The listing builds one solid part. Answer for the finished solid, in the listing's coordinates (mm). A direction names the side the tool comes from. Coordinates: 2 decimals unless noted, no trailing zeros. Order: outer loops, then holes, each group sorted by start corner. A loop starts at its lowest first (then second) coordinate and runs counter-clockwise, first axis right, second up. Notation, with made-up numbers: (-14, -24.5) -> (21, -24.5) arc R17 ccw to (21, -7.5) -> close; hole circle Ø5 at (-20, -27.75). An arc over 180 degrees is marked (long way). Answer in a Markdown table with one row per item.
```python
from build123d import *

# Parameters (mm, degrees)
SKETCH1_R                = 37.5
BOSS_EXTRUDE1_DEPTH      = 12
SKETCH2_R                = 30
BOSS_EXTRUDE2_DEPTH      = 56
BOSS_EXTRUDE3_DEPTH      = 5
BOSS_EXTRUDE3_DEPTH_BACK = 1
SKETCH4_W                = 75
SKETCH4_H                = 15
SKETCH4_R                = 3.5
MOVE_FACE3_BY            = 10
MOVE_FACE3_2_BY          = 10
BOSS_EXTRUDE4_DEPTH      = 12
BOSS_EXTRUDE5_DEPTH      = 68
MOVE_START               = 42.5
MOVE_FACE1_OUTLINE_W     = 95
MOVE_FACE1_OUTLINE_H     = 83
MOVE_FACE1_OUTLINE_R     = 3.5
MOVE_FACE1_DEPTH         = 10
SKETCH11_W               = 95
SKETCH11_H               = 15
BOSS_EXTRUDE7_DEPTH      = 20
CUT_EXTRUDE1_DEPTH       = 103.720494547
CUT_EXTRUDE1_DEPTH_BACK  = 103.720494547
SKETCH12_R               = 2.5
SKETCH13_R               = 6.5
CUT_EXTRUDE2_DEPTH       = 5
MOVE_FACE2_BY            = 7
DELETEFACE1_START        = -20
DELETEFACE1_OUTLINE_W    = 95
DELETEFACE1_OUTLINE_H    = 8
DELETEFACE1_DEPTH        = 20
CUT_EXTRUDE3_DEPTH       = 103.359660059
CUT_EXTRUDE3_DEPTH_BACK  = 3
SKETCH15_R               = 2
CUT_EXTRUDE4_DEPTH       = 96.818839484
MOVE_FACE4_BY            = 20
SKETCH16_W               = 55
SKETCH16_H               = 35
CUT_EXTRUDE5_DEPTH       = 10
SKETCH17_W               = 20
SKETCH17_H               = 50
CUT_EXTRUDE6_DEPTH       = 5
SKETCH18_R               = 2
CUT_EXTRUDE7_DEPTH       = 114.535236825
SKETCH19_R               = 2.5
CUT_EXTRUDE8_DEPTH       = 114.781589028


# Read off the part's stored shape, not the designer's step: Move Face1, DeleteFace1
with BuildPart() as part:
    # Sketch1 → Boss-Extrude1 (new body)
    with BuildSketch(Plane(origin=(0, 0, 0), x_dir=(1, 0, 0), z_dir=(0, 1, 0))):
        with Locations(Location((0, 0, 0), (0, 0, 270))):
            Circle(SKETCH1_R)
    extrude(amount=BOSS_EXTRUDE1_DEPTH)

    # Sketch2 → Boss-Extrude2 (add)
    with BuildSketch(Plane(origin=(0, 12, 0), x_dir=(1, 0, 0), z_dir=(0, 1, 0))):
        with Locations(Location((0, 0, 0), (0, 0, 270))):
            Circle(SKETCH2_R)
    extrude(amount=BOSS_EXTRUDE2_DEPTH)


with BuildPart() as body_2:
    # Sketch4 → Boss-Extrude3 (new, two sides: drawn at the far end of the back side and taken through both)
    with BuildSketch(Plane.XY.offset(37.5).offset(-BOSS_EXTRUDE3_DEPTH_BACK)):
        with Locations((0, 75.5)):
            Rectangle(SKETCH4_W, SKETCH4_H)
        with Locations((0, 76)):
            Circle(SKETCH4_R, mode=Mode.SUBTRACT)
    extrude(amount=BOSS_EXTRUDE3_DEPTH + BOSS_EXTRUDE3_DEPTH_BACK)

    # Move Face3: a face moved outward by 10.0
    extrude(body_2.faces().sort_by_distance((-37.5, 75.5, 39.5))[0], amount=MOVE_FACE3_BY, dir=(-1, 0, 0))

    # Move Face3 2: a face moved outward by 10.0
    extrude(body_2.faces().sort_by_distance((37.5, 75.5, 39.5))[0], amount=MOVE_FACE3_2_BY, dir=(1, 0, 0))



with BuildPart() as body_3:
    # Sketch6 → Boss-Extrude4 (new body)
    with BuildSketch(Plane.XZ):
        with BuildLine():
            Line((42.5, 0), (37.5, 0))
            ThreePointArc((37.5, 0), (0, 37.5), (-37.5, 0))
            Line((-37.5, 0), (-42.5, 0))
            ThreePointArc((-42.5, 0), (0, 42.5), (42.5, 0))
        make_face()
    extrude(amount=-BOSS_EXTRUDE4_DEPTH)


with BuildPart() as body_2_1:
    add(body_2.part)

    add(body_3.part)  # Boss-Extrude5 merges body 3
    # Sketch7 → Boss-Extrude5 (add)
    with BuildSketch(Plane.XZ.offset(-68)):
        with BuildLine():
            Line((8.602325267, 36.5), (47.5, 36.5))
            Line((47.5, 36.5), (47.5, 42.5))
            Line((47.5, 42.5), (-47.5, 42.5))
            Line((-47.5, 42.5), (-47.5, 36.5))
            Line((-47.5, 36.5), (-8.602325267, 36.5))
            ThreePointArc((-8.602325267, 36.5), (0, 37.5), (8.602325267, 36.5))
        make_face()
    extrude(amount=BOSS_EXTRUDE5_DEPTH)

    # Move Face1 outline → Move Face1 (add)
    with BuildSketch(Plane.XY.offset(MOVE_START)):
        with Locations((0, 41.5)):
            Rectangle(MOVE_FACE1_OUTLINE_W, MOVE_FACE1_OUTLINE_H)
        with Locations((0, 76)):
            Circle(MOVE_FACE1_OUTLINE_R, mode=Mode.SUBTRACT)
    extrude(amount=MOVE_FACE1_DEPTH)

    # Sketch11 → Boss-Extrude7 (add)
    with BuildSketch(Plane.XZ):
        with Locations((0, 45)):
            Rectangle(SKETCH11_W, SKETCH11_H)
    extrude(amount=BOSS_EXTRUDE7_DEPTH)

    # Sketch12 → Cut-Extrude1 (cut, two sides: drawn at the far end of the back side and taken through both)
    with BuildSketch(Plane(origin=(0, 0, 37.5), x_dir=(-1, 0, 0), z_dir=(0, 0, -1)).offset(-CUT_EXTRUDE1_DEPTH_BACK)):
        with Locations((-15, 20)):
            Circle(SKETCH12_R)
        with Locations((15, 20)):
            Circle(SKETCH12_R)
        with Locations((-15, 50)):
            Circle(SKETCH12_R)
        with Locations((15, 50)):
            Circle(SKETCH12_R)
    extrude(amount=CUT_EXTRUDE1_DEPTH + CUT_EXTRUDE1_DEPTH_BACK, mode=Mode.SUBTRACT)

    # Sketch13 → Cut-Extrude2 (cut)
    with BuildSketch(Plane(origin=(0, 0, 36.5), x_dir=(-1, 0, 0), z_dir=(0, 0, -1))):
        with Locations((-15, 50)):
            Circle(SKETCH13_R)
        with Locations((15, 50)):
            Circle(SKETCH13_R)
        with Locations((-15, 20)):
            Circle(SKETCH13_R)
        with Locations((15, 20)):
            Circle(SKETCH13_R)
    extrude(amount=-CUT_EXTRUDE2_DEPTH, mode=Mode.SUBTRACT)

    # Move Face2: a face moved inward by 7.0
    extrude(body_2_1.faces().sort_by_distance((0, 31.294429556, 52.5))[0], amount=MOVE_FACE2_BY, dir=(0, 0, -1), mode=Mode.SUBTRACT)

    # DeleteFace1 outline → DeleteFace1 (cut)
    with BuildSketch(Plane(origin=(0, 0, 0), x_dir=(1, 0, 0), z_dir=(0, 1, 0)).offset(DELETEFACE1_START)):
        with Locations((0, -41.5)):
            Rectangle(DELETEFACE1_OUTLINE_W, DELETEFACE1_OUTLINE_H)
    extrude(amount=DELETEFACE1_DEPTH, mode=Mode.SUBTRACT)

    # Sketch14 → Cut-Extrude3 (cut, two sides: drawn at the far end of the back side and taken through both)
    with BuildSketch(Plane(origin=(0, 0, 36.5), x_dir=(-1, 0, 0), z_dir=(0, 0, -1)).offset(-CUT_EXTRUDE3_DEPTH_BACK)):
        Polygon((47.5, 0), (-42.5, 0), (-47.5, 0), (-47.5, 12), (-42.5, 12), (47.5, 12), align=None)
    extrude(amount=CUT_EXTRUDE3_DEPTH + CUT_EXTRUDE3_DEPTH_BACK, mode=Mode.SUBTRACT)

    # Sketch15 → Cut-Extrude4 (cut, through all)
    with BuildSketch(Plane(origin=(0, 0, 39.5), x_dir=(-1, 0, 0), z_dir=(0, 0, -1))):
        with Locations((44.5, 6)):
            Circle(SKETCH15_R)
        with Locations((-44.5, 6)):
            Circle(SKETCH15_R)
    extrude(amount=-CUT_EXTRUDE4_DEPTH, mode=Mode.SUBTRACT)

    # Move Face4: a face moved outward by 20.0
    extrude(body_2_1.faces().sort_by_distance((0, 83, 41))[0], amount=MOVE_FACE4_BY, dir=(0, 1, 0))

    # Sketch16 → Cut-Extrude5 (cut)
    with BuildSketch(Plane(origin=(0, 0, 36.5), x_dir=(-1, 0, 0), z_dir=(0, 0, -1))):
        with Locations((0, 85.5)):
            Rectangle(SKETCH16_W, SKETCH16_H)
    extrude(amount=-CUT_EXTRUDE5_DEPTH, mode=Mode.SUBTRACT)

    # Sketch17 → Cut-Extrude6 (cut)
    with BuildSketch(Plane(origin=(0, 0, 36.5), x_dir=(-1, 0, 0), z_dir=(0, 0, -1))):
        with Locations((37.5, 78)):
            Rectangle(SKETCH17_W, SKETCH17_H)
        with Locations((-37.5, 78)):
            Rectangle(SKETCH17_W, SKETCH17_H)
    extrude(amount=-CUT_EXTRUDE6_DEPTH, mode=Mode.SUBTRACT)

    # Sketch18 → Cut-Extrude7 (cut, through all)
    with BuildSketch(Plane(origin=(0, 0, 41.5), x_dir=(-1, 0, 0), z_dir=(0, 0, -1))):
        with Locations((-42.5, 58)):
            Circle(SKETCH18_R)
        with Locations((-42.5, 100)):
            Circle(SKETCH18_R)
        with Locations(Location((42.5, 100, 0), (0, 0, 180))):
            Circle(SKETCH18_R)
        with Locations(Location((42.5, 58, 0), (0, 0, 180))):
            Circle(SKETCH18_R)
    extrude(amount=-CUT_EXTRUDE7_DEPTH, mode=Mode.SUBTRACT)

    # Sketch19 → Cut-Extrude8 (cut, through all)
    with BuildSketch(Plane.XY.offset(45.5)):
        with Locations((0, 35)):
            Circle(SKETCH19_R)
    extrude(amount=-CUT_EXTRUDE8_DEPTH, mode=Mode.SUBTRACT)


solid = body_2_1.part
```
(1) A cutting plane is placed at A-A, the plane y = 35. Determine the outline of the cut face in (x, z).
Check values:
| item | result |
|---|---|
| outline | (-47.5, 36.5) -> (-8.6, 36.5) arc R37.5 cw to (-2.5, 37.42) -> (-2.5, 45.5) -> (-47.5, 45.5) -> close; (2.5, 37.42) arc R37.5 cw to (8.6, 36.5) -> (47.5, 36.5) -> (47.5, 45.5) -> (2.5, 45.5) -> close |
(2) Find the intervals of material crossed by line 1 along Y through (x, z) = (-15, 43.95); line 2 along X through (y, z) = (20, 43.2); line 3 along Y through (x, z) = (15, 39.45), in increasing order. Write a range as from..to.
Check values:
| item | result |
|---|---|
| line 1 | 0..17.5, 22.5..47.5, 52.5..68 |
| line 2 | -47.5..-17.5, -12.5..12.5, 17.5..47.5 |
| line 3 | 12..13.5, 26.5..43.5, 56.5..68 |
(3) For a pull along Y with two mould halves and no side action, classify faces 5 (the cylindrical face through (-12.5, 50.1, 43.5)), 6 (the flat face through (38, 53, 39)), 7 (the flat face through (-1, 12, 38)), 8 (the flat face through (-27.5, 60, 39)) as released by +Y, released by -Y, zero draft, split by the parting line, or undercut.
Check values:
| item | result |
|---|---|
| face 5 | undercut |
| face 6 | released by +Y |
| face 7 | released by -Y |
| face 8 | zero draft |
(4) Which of the six approach directions +Z, -Z, +X, -X, +Y, -Y give full straight-line access (tool end or side, diameter ignored) to faces 1 (the flat face through (-37, 53, 39)), 2 (the flat face through (-18, 20, 41.5)), 3 (the flat face through (38, 78, 41.5)), 4 (the flat face through (0, 68, 41))?
Check values:
| item | result |
|---|---|
| face 1 | -Z, -X, +Y |
| face 2 | -Z |
| face 3 | -Z, +X, +Y |
| face 4 | +Z, -Z, +Y |
(5) Flat-ended cylindrical pins translate along their axes: pin 1 (1.5 mm diameter, centred on x = -40.5, z = 38.5, fed in from +Y); pin 2 (6.5 mm diameter, centred on x = 17.5, y = 50, fed in from -Z); pin 3 (4.5 mm diameter, centred on x = -15, y = 20, fed in from -Z); pin 4 (6.5 mm diameter, centred on x = 0, y = 35, fed in from -Z). Find the tip coordinate at first contact, or state that the pin passes through.
Check values:
| item | result |
|---|---|
| pin 1 | y = 53 |
| pin 2 | z = 41.5 |
| pin 3 | through |
| pin 4 | z = 37.36 |
(6) A cutting plane is placed at B-B, the plane x = 15. Determine the outline of the cut face in (y, z).
Check values:
| item | result |
|---|---|
| outline | (0, 39.5) -> (12, 39.5) -> (12, 36.5) -> (13.5, 36.5) -> (13.5, 41.5) -> (17.5, 41.5) -> (17.5, 45.5) -> (0, 45.5) -> close; (22.5, 41.5) -> (26.5, 41.5) -> (26.5, 36.5) -> (43.5, 36.5) -> (43.5, 41.5) -> (47.5, 41.5) -> (47.5, 45.5) -> (22.5, 45.5) -> close; (52.5, 41.5) -> (56.5, 41.5) -> (56.5, 36.5) -> (68, 36.5) -> (68, 45.5) -> (52.5, 45.5) -> close |
(7) A cutting plane is placed at C-C, the plane z = 43.75. Count the separate pieces of the cut face and the enclosed holes in it, then the cut area to 3 significant figures.
Check values:
| item | result |
|---|---|
| separate pieces | 1 |
| enclosed holes | 11 |
| area | 7,690 mm² |
(8) A cutting plane is placed at D-D, the plane y = 50. Determine the outline of the cut face in (x, z).
Check values:
| item | result |
|---|---|
| outline | (-47.5, 36.5) -> (-21.5, 36.5) -> (-21.5, 41.5) -> (-17.5, 41.5) -> (-17.5, 45.5) -> (-47.5, 45.5) -> close; (-12.5, 41.5) -> (-8.5, 41.5) -> (-8.5, 36.52) arc R37.5 cw to (8.5, 36.52) -> (8.5, 41.5) -> (12.5, 41.5) -> (12.5, 45.5) -> (-12.5, 45.5) -> close; (17.5, 41.5) -> (21.5, 41.5) -> (21.5, 36.5) -> (47.5, 36.5) -> (47.5, 45.5) -> (17.5, 45.5) -> close |
